from build123d import *

# Parameters (mm, degrees)
F1_DEPTH    = 5
F2_R        = 5
F3_R        = 5
F4_R        = 5
F5_R        = 5
F6_R        = 2.49999
F7_T1_DEPTH = 15.5


# Not quite as in the source:
# - a fillet or chamfer that OpenCascade refuses, or shapes differently, is made with other operations: its cross-section is extruded or revolved along the edge and cut away or added
# - a fillet or chamfer is up to 0.001 mm smaller than in the source, because OpenCascade refuses the exact size
# - ends of sketch curves that miss each other by under 0.0002 mm in the source are joined


with BuildPart() as f1:
    # F0 (on Front) → F1 (new body)
    with BuildSketch(Plane.XZ):
        with BuildLine():
            ThreePointArc((8.5340575526, 1.5524331459), (5.288604189, 4.5896124098), (1.5539747452, 7))
            Line((1.5539747452, 7), (0.4354276506, 7))
            ThreePointArc((0.4354276506, 7), (3.7532215697, 5.0934578086), (6.7313555625, 2.6906724375))
            ThreePointArc((6.7313555625, 2.6906724375), (7.6907583635, 2.2142400773), (8.526661649, 1.544383954))
            Line((8.526661649, 1.544383954), (8.5340575526, 1.5524331459))
        make_face()
        with BuildLine():
            Line((0.4354276506, 7), (1.5539747452, 7))
            ThreePointArc((1.5539747452, 7), (0.9960319704, 7.2841112302), (0.4311083103, 7.5540752821))
            ThreePointArc((0.4311083103, 7.5540752821), (0.1227273169, 7.4207378189), (-0.1837962437, 7.2831841097))
            ThreePointArc((-0.1837962437, 7.2831841097), (0.1268056153, 7.1437566434), (0.4354276506, 7))
        make_face()
        with BuildLine():
            ThreePointArc((-0.1837962437, 7.2831841097), (0.1227273169, 7.4207378189), (0.4311083103, 7.5540752821))
            ThreePointArc((0.4311083103, 7.5540752821), (0.1226739578, 7.6941799666), (-0.1876416897, 7.830066947))
            ThreePointArc((-0.1876416897, 7.830066947), (-0.4960575858, 7.6899267332), (-0.8025462438, 7.5456202987))
            ThreePointArc((-0.8025462438, 7.5456202987), (-0.4922657174, 7.4165371782), (-0.1837962437, 7.2831841097))
        make_face()
        with BuildLine():
            ThreePointArc((9.8891323912, -0.952916211), (9.474622014, 0.231088934), (8.7784454506, 1.2746526497))
            ThreePointArc((8.7784454506, 1.2746526497), (8.6550425686, 1.4118417052), (8.526661649, 1.544383954))
            Line((8.526661649, 1.544383954), (8.1941180403, 1.1824664061))
            ThreePointArc((8.1941180403, 1.1824664061), (8.2977627182, 1.0651806637), (8.4006513445, 0.9472311186))
            ThreePointArc((8.4006513445, 0.9472311186), (9.1684512833, 0.0156127298), (9.8891323912, -0.952916211))
        make_face()
        with BuildLine():
            ThreePointArc((-5.7758389138, 3.7449434933), (-3.3782514437, 5.5249211523), (-0.7819293264, 7))
            Line((-0.7819293264, 7), (-1.874342087, 7))
            ThreePointArc((-1.874342087, 7), (-4.0392081747, 5.6857592036), (-6.0600011216, 4.1592370405))
            Line((-6.0600011216, 4.1592370405), (-5.7758389138, 3.7449434933))
        make_face()
        with BuildLine():
            Line((-1.874342087, 7), (-0.7819293264, 7))
            ThreePointArc((-0.7819293264, 7), (-0.4838189836, 7.143611709), (-0.1837962437, 7.2831841097))
            ThreePointArc((-0.1837962437, 7.2831841097), (-0.4922657174, 7.4165371782), (-0.8025462438, 7.5456202987))
            ThreePointArc((-0.8025462438, 7.5456202987), (-1.341725683, 7.2792562383), (-1.874342087, 7))
        make_face()
        with BuildLine():
            ThreePointArc((8.526661649, 1.544383954), (7.6907583635, 2.2142400773), (6.7313555625, 2.6906724375))
            ThreePointArc((6.7313555625, 2.6906724375), (7.4790116412, 1.9523538866), (8.1941180403, 1.1824664061))
            Line((8.1941180403, 1.1824664061), (8.526661649, 1.544383954))
        make_face()
        with BuildLine():
            ThreePointArc((5, -7), (8.5355339059, -5.5355339059), (10, -2))
            ThreePointArc((10, -2), (9.9722058463, -1.4735315565), (9.8891323912, -0.952916211))
            ThreePointArc((9.8891323912, -0.952916211), (9.1684512833, 0.0156127298), (8.4006513445, 0.9472311186))
            ThreePointArc((8.4006513445, 0.9472311186), (9.2162011355, -0.4272164851), (9.5, -2))
            ThreePointArc((9.5, -2), (8.1819805153, -5.1819805153), (5, -6.5))
            Line((5, -6.5), (5, -7))
        make_face()
        with BuildLine():
            Line((4.8047364689, -6.5), (2.8205505282, -6.5))
            ThreePointArc((2.8205505282, -6.5), (3.7870014268, -6.8506323775), (4.8047364689, -6.9961857605))
            Line((4.8047364689, -6.9961857605), (4.8047364689, -6.5))
        make_face()
        with BuildLine():
            ThreePointArc((4.8047364689, -6.9961857605), (3.7870014268, -6.8506323775), (2.8205505282, -6.5))
            Line((2.8205505282, -6.5), (-4.0635083269, -6.5))
            ThreePointArc((-4.0635083269, -6.5), (-5, -6.8729833462), (-6, -7))
            Line((-6, -7), (4.8047364689, -7))
            Line((4.8047364689, -7), (4.8047364689, -6.9961857605))
        make_face()
        with BuildLine():
            ThreePointArc((8.4006513445, 0.9472311186), (8.2977627182, 1.0651806637), (8.1941180403, 1.1824664061))
            Line((8.1941180403, 1.1824664061), (8.1880677147, 1.1758816487))
            ThreePointArc((8.1880677147, 1.1758816487), (8.2963182158, 1.0633782366), (8.4006513445, 0.9472311186))
        make_face()
        with BuildLine():
            ThreePointArc((4.8047364689, -6.9961857605), (4.9023496096, -6.9990463492), (5, -7))
            Line((5, -7), (5, -6.5))
            Line((5, -6.5), (4.8047364689, -6.5))
            Line((4.8047364689, -6.5), (4.8047364689, -6.9961857605))
        make_face()
        with BuildLine():
            ThreePointArc((-6, -7), (-5, -6.8729833462), (-4.0635083269, -6.5))
            Line((-4.0635083269, -6.5), (-6, -6.5))
            Line((-6, -6.5), (-6, -7))
        make_face()
        with BuildLine():
            Line((-12.1979728804, -3.5), (-11.6333076528, -3.5))
            ThreePointArc((-11.6333076528, -3.5), (-11.4981121732, -3.2492054316), (-11.3600093633, -3))
            Line((-11.3600093633, -3), (-11.9317121995, -3))
            ThreePointArc((-11.9317121995, -3), (-12.0662587747, -3.2492458247), (-12.1979728804, -3.5))
        make_face()
        with BuildLine():
            ThreePointArc((-11.3600093633, -3), (-11.4981121732, -3.2492054316), (-11.6333076528, -3.5))
            Line((-11.6333076528, -3.5), (-10, -3.5))
            Line((-10, -3.5), (-10, -3))
            Line((-10, -3), (-11.3600093633, -3))
        make_face()
        with BuildLine():
            ThreePointArc((-9.9686269666, -3.5), (-9.9921490369, -3.2504916502), (-10, -3))
            Line((-10, -3), (-10, -3.5))
            Line((-10, -3.5), (-9.9686269666, -3.5))
        make_face()
        with BuildLine():
            Line((-9.5, -3), (-10, -3))
            ThreePointArc((-10, -3), (-9.9921490369, -3.2504916502), (-9.9686269666, -3.5))
            Line((-9.9686269666, -3.5), (-9.4641016151, -3.5))
            ThreePointArc((-9.4641016151, -3.5), (-9.491013868, -3.2506435188), (-9.5, -3))
        make_face()
        with BuildLine():
            ThreePointArc((-9.9686269666, -3.5), (-8.6457513111, -6), (-6, -7))
            Line((-6, -7), (-6, -6.5))
            ThreePointArc((-6, -6.5), (-8.2912878475, -5.6457513111), (-9.4641016151, -3.5))
            Line((-9.4641016151, -3.5), (-9.9686269666, -3.5))
        make_face()
        with BuildLine():
            Line((-15, -3.5), (-12.1979728804, -3.5))
            ThreePointArc((-12.1979728804, -3.5), (-12.0662587747, -3.2492458247), (-11.9317121995, -3))
            Line((-11.9317121995, -3), (-15, -3))
            Line((-15, -3), (-15, -3.5))
        make_face()
    extrude(amount=F1_DEPTH)

    # F2
    f2_edges = [f1.edges().sort_by_distance(p)[0] for p in [
        (-9.968627, -2.5, -3.5),
    ]]
    fillet(f2_edges, radius=F2_R)

    # F3
    f3_edges = [f1.edges().sort_by_distance(p)[0] for p in [
        (-9.5, -2.5, -3),
    ]]
    fillet(f3_edges, radius=F3_R)

    # F4
    f4_edges = [f1.edges().sort_by_distance(p)[0] for p in [
        (-0.183796, -2.5, 7.283184),
    ]]
    fillet(f4_edges, radius=F4_R)

    # F5
    f5_edges = [f1.edges().sort_by_distance(p)[0] for p in [
        (-0.187642, -2.5, 7.830067),
    ]]
    fillet(f5_edges, radius=F5_R)

    # F6 (radius 2.5 in the source; OpenCascade refuses exactly that, so slightly less here)
    f6_edges = [f1.edges().sort_by_distance(p)[0] for p in [
        (-5.91792, -5, 3.95209),
        (-5.91792, 0, 3.95209),
    ]]
    fillet(f6_edges, radius=F6_R)

    # F7: fillet of radius 3 on 2 edges, made by hand

    # F7_s2 → F7_t1 (cut)
    with BuildSketch(Plane.XY.offset(-11)):
        with BuildLine():
            ThreePointArc((-15, -2), (-14.1213203436, -4.1213203436), (-12, -5))
            Line((-12, -5), (-15, -5))
            Line((-15, -5), (-15, -2))
        make_face()
        with BuildLine():
            ThreePointArc((-12, 0), (-14.1213203436, -0.8786796564), (-15, -3))
            Line((-15, -3), (-15, 0))
            Line((-15, 0), (-12, 0))
        make_face()
    extrude(amount=F7_T1_DEPTH, mode=Mode.SUBTRACT)


solid = f1.part
Can you work these out from the model? Positions are in its coordinate system, mm. A direction names the side the tool comes from. Round coordinates to 2 decimals unless told otherwise and drop trailing zeros. Write each loop counter-clockwise with the first axis right and the second up, starting at its lowest first coordinate (ties: lowest second). Pieces come first, ordered by that corner, then holes. Notation, with made-up numbers: (74, -10) - (132, -10) arc R37 cw to (132, 26) - close; hole circle Ø8 at (37.5, 46.25). An arc over 180 degrees is marked (long way). Write each question's results on one line, items separated by ' | '. Start each with the question number.
1) Suppose I cut it at D-D (x = -8.25). List the corners of the cut face in (y, z) for me.
2) We'd pull the mould along X, two halves only. Please class faces 5 (the flat face through (-14, -2, -3.5)), 6 (the cylindrical face through (8.217, -2.465, -5.147)), 7 (the cylindrical face through (-5.36, -4.25, 4.4)): released by +X, released by -X, zero draft, split by the parting line, or undercut.
3) Suppose I cut it at C-C (z = 0.25). List the corners of the cut face in (x, y) for me.
4) For pin 1 Ø1.7 at (x, y) = (-13.5, -1.5) entering from +Z; pin 2 Ø1.5 at (x, y) = (-14, -3) entering from -Z; pin 3 Ø1.5 at (x, z) = (-12, -2) entering from -Y, each with a flat end and sliding along its axis, tell me the tip position at first contact or that it passes through.
5) Suppose I cut it at A-A (x = 2.75). List the corners of the cut face in (y, z) for me, and give its area (3 significant figures).
6) Which directions (+Z, -Z, +X, -X, +Y, -Y) give clear straight access to the entire face, cutting with the end or side of a thin tool? Please do faces 1 (the flat face through (-14, -2, -3)), 2 (the cylindrical face through (9.21, -2.46, -0.41)), 3 (the cylindrical face through (-5.3, -0.7, 4.4)), 4 (the cylindrical face through (-3.986, -2.465, 5.116)).
7) Suppose I cut it at B-B (z = -6). List the corners of the cut face in (x, y) for me, and give its area (3 significant figures).
8) Please list where these lines run through material, in increasing order: line 1 (Z direction, x = 5.25, y = -3.55); line 2 (Z direction, x = 4, y = -4.6); line 3 (X direction, y = -0.65, z = 6.25).
Here are the results:
1) outline: (-5, -6.31) - (0, -6.31) - (0, -5.68) - (-5, -5.68) - close
2) face 5: zero draft | face 6: undercut | face 7: released by -X
3) outline: (8.9, -5) - (9.47, -5) - (9.47, 0) - (8.9, 0) - close
4) pin 1: stops at z = -3 | pin 2: stops at z = -3.5 | pin 3: passes through
5) outline: (-5, -7) - (0, -7) - (0, -6.5) - (-5, -6.5) - close; (-5, 5.74) - (0, 5.74) - (0, 6.33) - (-5, 6.33) - close | area: 5.42 mm2
6) face 1: +Z, -X, +Y, -Y | face 2: -X, +Y, -Y | face 3: -X, +Y | face 4: +Y, -Y
7) outline: (-8.65, -5) - (-7.8, -5) - (-7.8, 0) - (-8.65, 0) - close; (7.06, -5) - (8, -5) - (8, 0) - (7.06, 0) - close | area: 8.91 mm2
8) line 1: z = -6.99 to -6.49, 3.98 to 4.62 | line 2: z = -7 to -6.5, 4.92 to 5.53 | line 3: x = -3.17 to -2.11, 1.82 to 2.88
